Source: CAD feature listing. Evaluate the final solid. Frame: model axes, mm. Give positions to 0.01 mm unless a question says otherwise; leave off trailing zeros. Write each loop counter-clockwise with the first axis right and the second up, starting at its lowest first coordinate (ties: lowest second). Pieces come first, ordered by that corner, then holes. Notation, with made-up numbers: (34.25, 22.5) - (76.25, 22.5) arc R9 cw to (76.25, 35.5) - close; hole circle Ø6 at (-7.5, -40). An arc over 180 degrees is marked (long way). One line per question, with ' | ' between items. Start each with the question number.
(1) Section A-A, the plane x = -12.7. Return loops of the section in (y, z).
(2) Ray query, line 1 (Y direction, x = 6, z = 0.75); line 2 (Y direction, x = -38.1, z = 0.9); line 3 (Y direction, x = -52.5, z = 1.25). Return the intervals inside material, ascending. Write a range as [from, to].
(3) Section D-D, the plane x = -44.45. Return loops of the section in (y, z).
(4) Section C-C, the plane z = 0.65. State how many separate pieces and enclosed holes the cut face has, plus the area to 3 significant figures.
(5) Draft query along X for faces 1 (the cylindrical face through (9.75, 62.07, 0.8)), 2 (the cylindrical face through (-19.32, 60.83, 0.8)). Return one class per face: +X half, -X half, draft (parallel to the pull), parting line (faces both ways), or undercut.
(6) Section B-B, the plane y = 45. Return loops of the section in (x, z), plus the area to 3 significant figures.
Autodesk Inventor part; units mm, degrees
ref_plane "YZ Plane" through (0, 0, 0) normal (1, 0, 0) x (0, 1, 0)
ref_plane "XZ Plane" through (0, 0, 0) normal (0, 1, 0) x (-1, 0, 0)
ref_plane "XY Plane" through (0, 0, 0) normal (0, 0, 1) x (1, 0, 0)
sketch "Sketch1" plane through (0, 0, 0) normal (0, 0, 1) x (1, 0, 0)
  line L0 (57.15, -58.7375) -> (-57.15, -58.7375)
  line L1 (-57.15, -58.7375) -> (-57.15, 58.7375)
  line L2 (-57.15, 58.7375) -> (57.15, 58.7375)
  line L3 (57.15, 58.7375) -> (57.15, -58.7375)
  line L4 (57.15, -58.7375) -> (-57.15, 58.7375) construction
  line L5 (-57.15, -58.7375) -> (57.15, 58.7375) construction
  line L6 (-57.15, 58.7375) -> (-19.05, 58.7375)
  line L7 (-19.05, 58.7375) -> (-19.05, 20.6375)
  line L8 (-19.05, 20.6375) -> (-57.15, 20.6375)
  line L9 (-57.15, 20.6375) -> (-57.15, 58.7375)
  circle A0 centre (-38.1, 39.6875) radius 19.05
  circle A1 centre (-57.15, 58.7375) radius 4.7625
  circle A2 centre (57.15, 58.7375) radius 4.7625
  line L10 (-57.15, -58.7375) -> (-61.9125, -58.7375)
  line L11 (-61.9125, -58.7375) -> (-61.9125, 58.7375)
  line L12 (57.15, -58.7375) -> (61.9125, -58.7375)
  line L13 (61.9125, -58.7375) -> (61.9125, 58.7375)
  line L14 (57.15, 63.5) -> (-57.15, 63.5)
  circle A3 centre (-38.1, 39.6875) radius 10.9855
  circle A4 centre (-57.15, 58.7375) radius 2.1082
  circle A5 centre (57.15, 58.7375) radius 2.1082
  point P0 (0, 0)
  dimension "d0" = 114.3
  dimension "d1" = 117.475
  dimension "d2" = 38.1
  dimension "d3" = 38.1
  dimension "d4" = 9.525
  dimension "d5" = 9.525
  dimension "d6" = 4.7625
  dimension "d7" = 4.7625
  dimension "d8" = 21.971
  dimension "d9" = 4.2164
  dimension "d10" = 4.2164
extrude "Extrusion1" add sketch "Sketch1" along normal blind 1.5875 contours L0 L1 L8 L7 L2 A2 L3 | L3 A2 L13 L12 | L10 L11 A1 L1 | A2 L2 A5 L3 | L3 A5 L2 A2 | L1 A0 L8 | L2 A1 L14 A2 | L1 A1 L2 A0 | A0 | A0 L7 L8 | A1 L2 A4 L1 | L7 A0 L2 | L1 A4 L2 A1
sketch "Sketch2" plane through (0, 0, 1.5875) normal (0, 0, 1) x (1, 0, 0)
  circle A0 centre (-38.1, 39.6875) radius 10.9855
  line L0 (-38.1, 39.6875) -> (61.9125, 39.6875)
  line L1 (61.9125, -58.7375) -> (61.9125, 58.7375)
  circle A1 centre (-38.1, 39.6875) radius 6.35
  circle A2 centre (-12.7, 39.6875) radius 19.05
  circle A3 centre (38.1, 39.6875) radius 31.75
  circle A4 centre (-12.7, 39.6875) radius 10.9855
  circle A5 centre (38.1, 39.6875) radius 10.9855
  line L2 (-61.9125, 58.7375) -> (-61.9125, -58.7375)
  line L3 (-61.9125, -3.9688) -> (61.9125, -3.9688)
  line L4 (-38.1, 39.6875) -> (-12.7, 39.6875)
  line L5 (-25.4, 39.6875) -> (-25.4, -3.9688)
  circle A6 centre (-25.4, -3.9688) radius 10.9855
  line L6 (57.15, 63.5) -> (-57.15, 63.5)
  line L7 (-61.9125, -58.7375) -> (61.9125, -58.7375)
  line L8 (0, -58.7375) -> (0, 63.5)
  circle A7 centre (0, -46.0375) radius 19.05
  circle A8 centre (0, -46.0375) radius 2.1082
  point P0 (0, 0)
  dimension "d13" = 12.7
  dimension "d14" = 38.1
  dimension "d15" = 63.5
  dimension "d16" = 21.971
  dimension "d17" = 21.971
  dimension "d18" = 43.6562
  dimension "d19" = 21.971
  dimension "d20" = 25.4
  dimension "d21" = 38.1
  dimension "d22" = 12.7
  dimension "d23" = 4.2164
extrude "Extrusion2" cut sketch "Sketch2" against normal blind 1.5875 contours A4 L0 | L0 A4 | A6 L3 L5 | L5 L3 A6 | A5 L0 | L0 A5 | L3 A6 | A8 L8 | L8 A8
sketch "Sketch3" plane through (0, 0, 1.5875) normal (0, 0, 1) x (1, 0, 0)
  circle A0 centre (-25.4, -3.9688) radius 10.9855
  circle A1 centre (-38.1, 39.6875) radius 10.9855
  circle A2 centre (0, -46.0375) radius 2.1082
  circle A3 centre (0, -46.0375) radius 19.05
  circle A4 centre (-25.4, -3.9688) radius 19.05
  circle A5 centre (-38.1, 39.6875) radius 19.05
  circle A6 centre (-53.0324, 11.6681) radius 12.7
  circle A7 centre (-7.1902, -21.6764) radius 6.35
  circle A8 centre (-53.0324, 11.6681) radius 3.175
  circle A9 centre (-7.1902, -21.6764) radius 3.175
  point P0 (0, 0)
  dimension "d26" = 38.1
  dimension "d27" = 38.1
  dimension "d28" = 38.1
  dimension "d29" = 25.4
  dimension "d30" = 12.7
  dimension "d31" = 6.35
  dimension "d32" = 6.35
extrude "Extrusion3" cut sketch "Sketch3" against normal blind 25.4 contours A8 | A9
sketch "Sketch4" plane through (0, 0, 1.5875) normal (0, 0, 1) x (1, 0, 0)
  circle A0 centre (0, -46.0375) radius 2.1082
  line L0 (0, -46.0375) -> (-6.35, -46.0375)
  line L1 (-6.35, -46.0375) -> (-6.35, -39.6875)
  line L2 (-6.35, -39.6875) -> (0, -39.6875)
  line L3 (0, -39.6875) -> (0, -46.0375)
  circle A1 centre (-6.35, -39.6875) radius 2.1082
  line L4 (-61.9125, -58.7375) -> (61.9125, -58.7375)
  line L5 (-61.9125, 58.7375) -> (-61.9125, -58.7375)
  circle A2 centre (6.35, -39.6875) radius 2.1082
  circle A3 centre (19.05, -39.6875) radius 2.1082
  circle A4 centre (31.75, -39.6875) radius 2.1082
  circle A5 centre (44.45, -39.6875) radius 2.1082
  circle A6 centre (57.15, -39.6875) radius 2.1082
  circle A7 centre (-6.35, -52.3875) radius 2.1082
  circle A8 centre (6.35, -52.3875) radius 2.1082
  circle A9 centre (19.05, -52.3875) radius 2.1082
  circle A10 centre (31.75, -52.3875) radius 2.1082
  circle A11 centre (44.45, -52.3875) radius 2.1082
  circle A12 centre (57.15, -52.3875) radius 2.1082
  circle A13 centre (-19.05, -39.6875) radius 2.1082
  circle A14 centre (-31.75, -39.6875) radius 2.1082
  circle A15 centre (-44.45, -39.6875) radius 2.1082
  circle A16 centre (-57.15, -39.6875) radius 2.1082
  circle A17 centre (-6.35, -52.3875) radius 2.1082
  circle A18 centre (-19.05, -52.3875) radius 2.1082
  circle A19 centre (-31.75, -52.3875) radius 2.1082
  circle A20 centre (-44.45, -52.3875) radius 2.1082
  circle A21 centre (-57.15, -52.3875) radius 2.1082
  point P0 (0, 0)
  dimension "d35" = 6.35
  dimension "d36" = 6.35
  dimension "d37" = 4.2164
  dimension "d40" = 12.7
  dimension "d43" = 12.7
  dimension "d48" = 12.7
  dimension "d51" = 12.7
extrude "Extrusion4" cut sketch "Sketch4" against normal blind 25.4 contours A1 L1 L2 | L2 L1 A1 | A2 | A3 | A4 | A5 | A6 | A7 | A8 | A9 | A10 | A11 | A12 | A13 | A14 | A15 | A16 | A18 | A19 | A20 | A21
sketch "Sketch7" plane through (0, 0, 1.5875) normal (0, 0, 1) x (1, 0, 0)
  circle A0 centre (-12.7, 39.6875) radius 10.9855
  line L0 (12.7, 14.2875) -> (-38.1, 14.2875)
  line L1 (-38.1, 14.2875) -> (-38.1, 65.0875)
  line L2 (-38.1, 65.0875) -> (12.7, 65.0875)
  line L3 (12.7, 65.0875) -> (12.7, 14.2875)
  line L4 (12.7, 14.2875) -> (-38.1, 65.0875) construction
  line L5 (-38.1, 14.2875) -> (12.7, 65.0875) construction
  circle A1 centre (-38.1, 39.6875) radius 10.9855
  circle A2 centre (-57.15, 58.7375) radius 2.1082
  line L6 (-31.75, 20.6375) -> (6.35, 20.6375)
  line L7 (6.35, 20.6375) -> (6.35, 58.7375)
  line L8 (6.35, 58.7375) -> (-31.75, 58.7375)
  line L9 (-31.75, 58.7375) -> (-31.75, 20.6375)
  line L10 (-31.75, 20.6375) -> (6.35, 58.7375) construction
  line L11 (6.35, 20.6375) -> (-31.75, 58.7375) construction
  circle A3 centre (6.35, 58.7375) radius 2.1082
  circle A4 centre (6.35, 58.7375) radius 4.7625
  line L12 (11.1125, 58.7375) -> (11.1125, -58.7375)
  line L13 (-61.9125, -58.7375) -> (61.9125, -58.7375)
  line L14 (-61.9125, -58.7375) -> (61.9125, -58.7375)
  circle A5 centre (-25.4, -3.9688) radius 10.9855
  circle A6 centre (-25.4, -3.9688) radius 2.1082
  line L15 (-25.4, -3.9688) -> (-31.75, -3.9688)
  line L16 (-31.75, -3.9688) -> (-31.75, 2.3812)
  line L17 (-31.75, 2.3812) -> (-25.4, 2.3812)
  line L18 (-25.4, 2.3812) -> (-25.4, -3.9688)
  circle A7 centre (-31.75, 2.3812) radius 2.1082
  circle A8 centre (-38.1, -3.9688) radius 2.1082
  circle A9 centre (-50.8, -3.9688) radius 2.1082
  circle A10 centre (-12.7, -3.9688) radius 2.1082
  circle A11 centre (-25.4, -3.9688) radius 2.1082
  circle A12 centre (-38.1, -3.9688) radius 2.1082
  circle A13 centre (0, -3.9688) radius 2.1082
  circle A14 centre (-12.7, -3.9688) radius 2.1082
  circle A15 centre (-25.4, -3.9688) radius 2.1082
  circle A16 centre (-44.45, 2.3812) radius 2.1082
  circle A17 centre (-57.15, 2.3812) radius 2.1082
  circle A18 centre (-31.75, -10.3188) radius 2.1082
  circle A19 centre (-44.45, -10.3188) radius 2.1082
  circle A20 centre (-57.15, -10.3188) radius 2.1082
  circle A21 centre (-19.05, 2.3812) radius 2.1082
  circle A22 centre (-6.35, 2.3812) radius 2.1082
  circle A23 centre (6.35, 2.3812) radius 2.1082
  circle A24 centre (-31.75, -10.3188) radius 2.1082
  circle A25 centre (-19.05, -10.3188) radius 2.1082
  circle A26 centre (-6.35, -10.3188) radius 2.1082
  circle A27 centre (6.35, -10.3188) radius 2.1082
  line L19 (57.15, 63.5) -> (-57.15, 63.5)
  line L20 (61.9125, -58.7375) -> (61.9125, 58.7375)
  line L21 (11.1125, 58.7375) -> (61.9125, 58.7375)
  line L22 (61.9125, 58.7375) -> (61.9125, -58.7375)
  line L23 (61.9125, -58.7375) -> (11.1125, -58.7375)
  line L24 (11.1125, -58.7375) -> (11.1125, 58.7375)
  line L25 (61.9125, -58.7375) -> (61.9125, 58.7375)
  arc A28 (61.9125, 58.7375) -> (57.15, 63.5) centre (57.15, 58.7375) ccw
  point P0 (0, 0)
  point P1 (6.35, 63.5)
  dimension "d71" = 9.525
  dimension "d66" = 50.8
  dimension "d67" = 50.8
  dimension "d68" = 38.1
  dimension "d69" = 38.1
  dimension "d70" = 4.2164
  dimension "d72" = 4.2164
  dimension "d73" = 6.35
  dimension "d74" = 6.35
  dimension "d75" = 4.2164
  dimension "d78" = 12.7
  dimension "d81" = 12.7
  dimension "d86" = 12.7
  dimension "d89" = 12.7
  dimension "d94" = 12.7
  dimension "d97" = 12.7
extrude "Extrusion6" cut sketch "Sketch7" against normal blind 25.4 contours L3 L21 L20 L13 L12 L0 | L0 L12 L21 L3 | L21 A4 L19 L3 | L3 L19 A28 L21 | A3 L8 L7 | L7 L8 A3
sketch "Sketch9" plane through (0, 0, 1.5875) normal (0, 0, 1) x (1, 0, 0)
  circle A0 centre (0, -46.0375) radius 2.1082
  circle A1 centre (0, -46.0375) radius 2.1082
  line L0 (-61.9125, -58.7375) -> (11.1125, -58.7375)
  circle A2 centre (-12.7, -46.0375) radius 2.1082
  circle A3 centre (-25.4, -46.0375) radius 2.1082
  circle A4 centre (-38.1, -46.0375) radius 2.1082
  circle A5 centre (-50.8, -46.0375) radius 2.1082
  point P0 (0, 0)
  dimension "d117" = 12.7
extrude "Extrusion8" cut sketch "Sketch9" against normal blind 25.4
sketch "Sketch10" plane through (0, 0, 1.5875) normal (0, 0, 1) x (1, 0, 0)
  circle A0 centre (-12.7, 39.6875) radius 10.9855
  point P0 (0, 0)
extrude "Extrusion9" add sketch "Sketch10" against normal blind 1.5875
sketch "Sketch11" plane through (0, 0, 1.5875) normal (0, 0, 1) x (1, 0, 0)
  circle A0 centre (-25.4, -3.9688) radius 10.9855
  line L0 (-25.4, -3.9688) -> (-57.15, -3.9688)
  line L1 (-57.15, -3.9688) -> (-57.15, -10.3188)
  line L2 (-57.15, -10.3188) -> (-25.4, -10.3188)
  line L3 (-25.4, -10.3188) -> (-25.4, -3.9688)
  circle A1 centre (-57.15, -10.3188) radius 2.1082
  point P0 (0, 0)
  dimension "d126" = 31.75
  dimension "d127" = 6.35
  dimension "d128" = 4.2164
extrude "Extrusion10" cut sketch "Sketch11" against normal blind 1.5875 contours A1 L1 L2 | L2 L1 A1
sketch "Sketch12" plane through (0, 0, 1.5875) normal (0, 0, 1) x (1, 0, 0)
  circle A0 centre (-38.1, 39.6875) radius 10.9855
  line L0 (-57.15, 58.7375) -> (-19.05, 58.7375)
  line L1 (-19.05, 58.7375) -> (-19.05, 20.6375)
  line L2 (-19.05, 20.6375) -> (-57.15, 20.6375)
  line L3 (-57.15, 20.6375) -> (-57.15, 58.7375)
  line L4 (-57.15, 58.7375) -> (-19.05, 20.6375) construction
  line L5 (-19.05, 58.7375) -> (-57.15, 20.6375) construction
  circle A1 centre (-19.05, 58.7375) radius 2.1082
  circle A2 centre (-19.05, 20.6375) radius 2.1082
  point P0 (0, 0)
  dimension "d131" = 38.1
  dimension "d132" = 38.1
  dimension "d133" = 4.2164
  dimension "d134" = 4.2164
extrude "Extrusion11" cut sketch "Sketch12" against normal blind 1.5875 contours A1 L1 L0 | L0 L1 A1 | A2 L1 L2 | L2 L1 A2
sketch "Sketch13" plane through (0, 0, 1.5875) normal (0, 0, 1) x (1, 0, 0)
  circle A0 centre (-25.4, -3.9688) radius 10.9855
  line L0 (-25.4, -3.9688) -> (6.35, -3.9688)
  line L1 (6.35, -3.9688) -> (6.35, 2.3812)
  line L2 (6.35, 2.3812) -> (-25.4, 2.3812)
  line L3 (-25.4, 2.3812) -> (-25.4, -3.9688)
  circle A1 centre (6.35, 2.3812) radius 2.1082
  point P0 (0, 0)
  dimension "d137" = 31.75
  dimension "d138" = 6.35
  dimension "d139" = 4.2164
extrude "Extrusion12" cut sketch "Sketch13" against normal blind 1.5875 contours A1 L1 L2 | L2 L1 A1
properties part number "POM 1" material "Acetal Resin, Black"
Check sheet entries:
1) outline: (-58.74, 0) - (-48.15, 0) - (-48.15, 1.59) - (-58.74, 1.59) - close; (-43.93, 0) - (63.5, 0) - (63.5, 1.59) - (-43.93, 1.59) - close
2) line 1: [-58.74, -54.47], [-50.31, -41.77], [-37.61, 0.3], [4.46, 56.66], [60.82, 63.5] | line 2: [-58.74, -48.15], [-43.93, 28.7], [50.67, 63.5] | line 3: [-58.74, -47.28], [-44.79, 8.54], [14.8, 63.5]
3) outline: (-58.74, 0) - (-54.5, 0) - (-54.5, 1.59) - (-58.74, 1.59) - close; (-50.28, 0) - (-41.8, 0) - (-41.8, 1.59) - (-50.28, 1.59) - close; (-37.58, 0) - (30.72, 0) - (30.72, 1.59) - (-37.58, 1.59) - close; (48.65, 0) - (63.5, 0) - (63.5, 1.59) - (48.65, 1.59) - close
4) separate pieces: 1 | enclosed holes: 27 | area: 7,770 mm²
5) face 1: +X half | face 2: undercut
6) outline: (-61.91, 0) - (-47.72, 0) - (-47.72, 1.59) - (-61.91, 1.59) - close; (-28.48, 0) - (11.11, 0) - (11.11, 1.59) - (-28.48, 1.59) - close | area: 85.4 mm²
